Drawing for the job (mm, zero at the part's lowest x, y, z). Coordinates: 2 decimals unless noted, no trailing zeros. Order: outer loops, then holes, each group sorted by start corner. A loop starts at its lowest first (then second) coordinate and runs counter-clockwise, first axis right, second up. Notation, with made-up numbers: M 4.5,56 L 16.5,56 A21 ccw 16.5,66 Z; hole C 88.25,73.5 d7. An arc over 180 degrees is marked long. Write item = value, one per line. Start each with the question number.
Q1. Band-saw the part on B-B on x = 80.8. Write the cut outline in (y, z).
Q2. Drill centre lines: probe 1 along X at (y, z) = (6.25, 2.95); probe 2 along Y at (x, z) = (80.8, 3.35); probe 3 along X at (y, z) = (4, 1.75). Where is each one in solid material? Low to high.
Q3. Band-saw the part on C-C on z = 2.3. Write the cut outline in (x, y), plus the area to 3 significant figures.
Q4. Band-saw the part on A-A on y = 5. Write the cut outline in (x, z), plus the area to 3 significant figures.
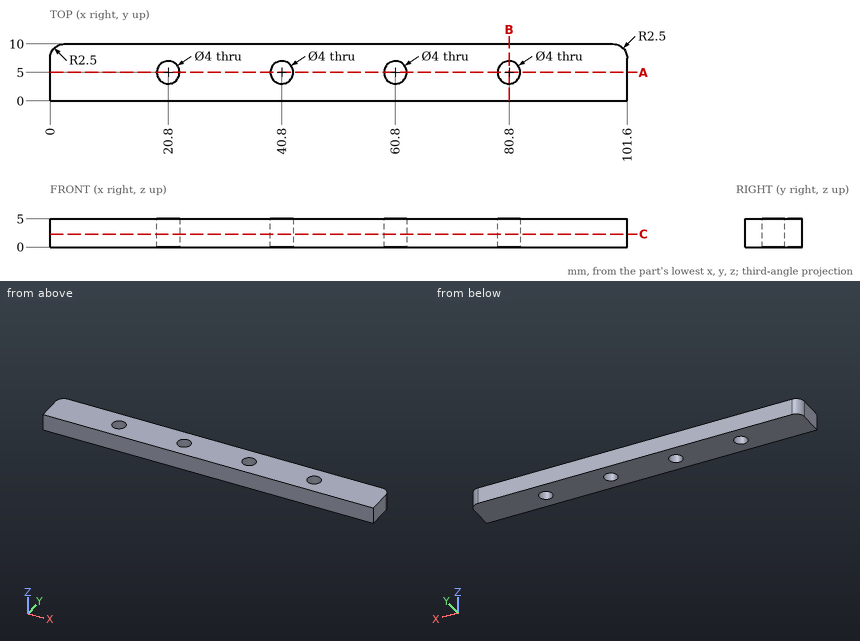
Recorded:
q1.outline = M 0,0 L 3,0 L 3,5 L 0,5 Z; M 7,0 L 10,0 L 10,5 L 7,5 Z
q2.probe_1 = 0 to 19.24, 22.36 to 39.24, 42.36 to 59.24, 62.36 to 79.24, 82.36 to 101.6
q2.probe_2 = 0 to 3, 7 to 10
q2.probe_3 = 0 to 19.07, 22.53 to 39.07, 42.53 to 59.07, 62.53 to 79.07, 82.53 to 101.6
q3.outline = M 0,0 L 101.6,0 L 101.6,7.5 A2.5 ccw 99.1,10 L 2.5,10 A2.5 ccw 0,7.5 Z; hole C 20.8,5 d4; hole C 40.8,5 d4; hole C 60.8,5 d4; hole C 80.8,5 d4
q3.area = 963 mm2
q4.outline = M 0,0 L 18.8,0 L 18.8,5 L 0,5 Z; M 22.8,0 L 38.8,0 L 38.8,5 L 22.8,5 Z; M 42.8,0 L 58.8,0 L 58.8,5 L 42.8,5 Z; M 62.8,0 L 78.8,0 L 78.8,5 L 62.8,5 Z; M 82.8,0 L 101.6,0 L 101.6,5 L 82.8,5 Z
q4.area = 428 mm2
